from build123d import *

# Parameters (mm, degrees)
EXTRUDE_1_DEPTH     = 2
SKETCH_7_OUTSIDE_W  = 58.13
SKETCH_7_OUTSIDE_H  = 88.13
CUT_EXTRUDE_5_DEPTH = 3
SKETCH_3_R          = 2.6
CUT_EXTRUDE_1_DEPTH = 3
FILLET_1_R          = 2.5


with BuildPart() as part:
    # Эскиз2 → Бобышка-Вытянуть1 (new body)
    with BuildSketch(Plane(origin=(0, 0, 0), x_dir=(1, 0, 0), z_dir=(0, 1, 0))):
        Polygon((33.713737203, -10), (33.713737203, 10), (25.042706268, 54.823619098), (5.724189742, 60), (-6.286262797, 15.176380902), (-6.286262797, -10), align=None)
    extrude(amount=EXTRUDE_1_DEPTH)

    # Эскиз7 outside → Вырез-Вытянуть5 (cut, through all)
    with BuildSketch(Plane(origin=(0, 2, 0), x_dir=(1, 0, 0), z_dir=(0, 1, 0))):
        with Locations((13.714, 25)):
            Rectangle(SKETCH_7_OUTSIDE_W, SKETCH_7_OUTSIDE_H)
        Polygon((32.213737203, -8.5), (32.213737203, 9.856246677), (23.748206001, 53.617565128), (6.784849914, 58.162882693), (-4.786262797, 14.978902156), (-4.786262797, -8.5), align=None, mode=Mode.SUBTRACT)
    extrude(amount=-CUT_EXTRUDE_5_DEPTH, mode=Mode.SUBTRACT)

    # Эскиз3 → Вырез-Вытянуть1 (cut, through all)
    with BuildSketch(Plane(origin=(0, 2, 0), x_dir=(1, 0, 0), z_dir=(0, 1, 0))):
        with Locations(Location((3.213737203, 0, 0), (0, 0, 270))):  # turned: the seam where the file's is
            Circle(SKETCH_3_R)
        with Locations(Location((7.748286174, 28.916997673, 0), (0, 0, 270))):  # turned: the seam where the file's is
            Circle(SKETCH_3_R)
        with Locations(Location((12.924667076, 48.235514199, 0), (0, 0, 270))):  # turned: the seam where the file's is
            Circle(SKETCH_3_R)
        with Locations(Location((23.213737203, 0, 0), (0, 0, 270))):  # turned: the seam where the file's is
            Circle(SKETCH_3_R)
        with Locations((43.213737203, 0)):
            Circle(SKETCH_3_R)
    extrude(amount=-CUT_EXTRUDE_1_DEPTH, mode=Mode.SUBTRACT)

    # Скругление1
    fillet_1_edges = [part.edges().sort_by_distance(p)[0] for p in [
        (6.784849914, 1, -58.162882693),
        (23.748206001, 1, -53.617565128),
        (32.213737203, 1, -9.856246677),
        (32.213737203, 1, 8.5),
        (-4.786262797, 1, 8.5),
        (-4.786262797, 1, -14.978902156),
    ]]
    fillet(fillet_1_edges, radius=FILLET_1_R)


solid = part.part
The listing builds one solid part. Answer for the finished solid, in the listing's coordinates (mm). Round coordinates to 2 decimals unless told otherwise and drop trailing zeros. Write each loop counter-clockwise with the first axis right and the second up, starting at its lowest first coordinate (ties: lowest second). Pieces come first, ordered by that corner, then holes. Notation, with made-up numbers: M -13,28 L 0,28 A19 ccw 0,63 Z; hole C -35,51.5 d11. An arc over 180 degrees is marked long. Write each question's results on one line, items separated by ' | '. Start each with the question number.
(1) The part is cut by section B-B, the plane x = 11.5. Write down the section's boundary in (y, z).
(2) The part is cut by section A-A, the plane z = 0. Write down the section's boundary in (x, y).
(3) The part is cut by section C-C, the plane z = -35.5. Write down the section's boundary in (x, y), and give its area (3 significant figures).
(4) Find the intervals of material crossed by line 1 (X direction, y = 0.5, z = 0); line 2 (Z direction, x = 22.5, y = 1.3); line 3 (Z direction, x = 22, y = 1.95), in increasing order.
(5) The part is cut by section D-D, the plane x = -1.5. Write down the section's boundary in (y, z).
(6) This flat-tipped pin is pushed along its axis until it touches: P1, Ø4.5, axis at x = 12.92, z = -48.24, coming from the +Y side. Where does it stop, or does it pass through?
(7) Determine the mould class of faces 1 (the cylindrical face through (31.46, 0.99, 7.79)), 2 (the cylindrical face through (5.44, 1.01, -27.72)), 3 (the flat face through (-4.786, 1, -4)) for opening direction Z: +Z half, -Z half, draft (parallel to the pull), parting line (faces both ways), or undercut.
Worked answers:
1) outline: M 0,-56.9 L 2,-56.9 L 2,-50.41 L 0,-50.41 Z; M 0,-46.06 L 2,-46.06 L 2,8.5 L 0,8.5 Z
2) outline: M -4.79,0 L 0.61,0 L 0.61,2 L -4.79,2 Z; M 5.81,0 L 20.61,0 L 20.61,2 L 5.81,2 Z; M 25.81,0 L 32.21,0 L 32.21,2 L 25.81,2 Z
3) outline: M 0.71,0 L 27.25,0 L 27.25,2 L 0.71,2 Z | area: 53.1 mm²
4) line 1: x = -4.79 to 0.61, 5.81 to 20.61, 25.81 to 32.21 | line 2: z = -53.94 to -2.5, 2.5 to 8.5 | line 3: z = -54.09 to -2.3, 2.3 to 8.5
5) outline: M 0,-27.24 L 2,-27.24 L 2,8.5 L 0,8.5 Z
6) P1: passes through
7) face 1: +Z half | face 2: undercut | face 3: draft
